Verification items for this drawing (mm, ordinates from the low corner). Round coordinates to 2 decimals unless told otherwise and drop trailing zeros. Loops run counter-clockwise (first coordinate to the right, second up) from the corner with the lowest first, then second, coordinate; pieces in that order, holes last. Notation, with made-up numbers: (31, 32.5) - (65, 32.5) arc R30 ccw to (65, 65.5) - close; hole circle Ø7 at (19.25, 17). An arc over 180 degrees is marked (long way). Put each result on its own line as item: value.
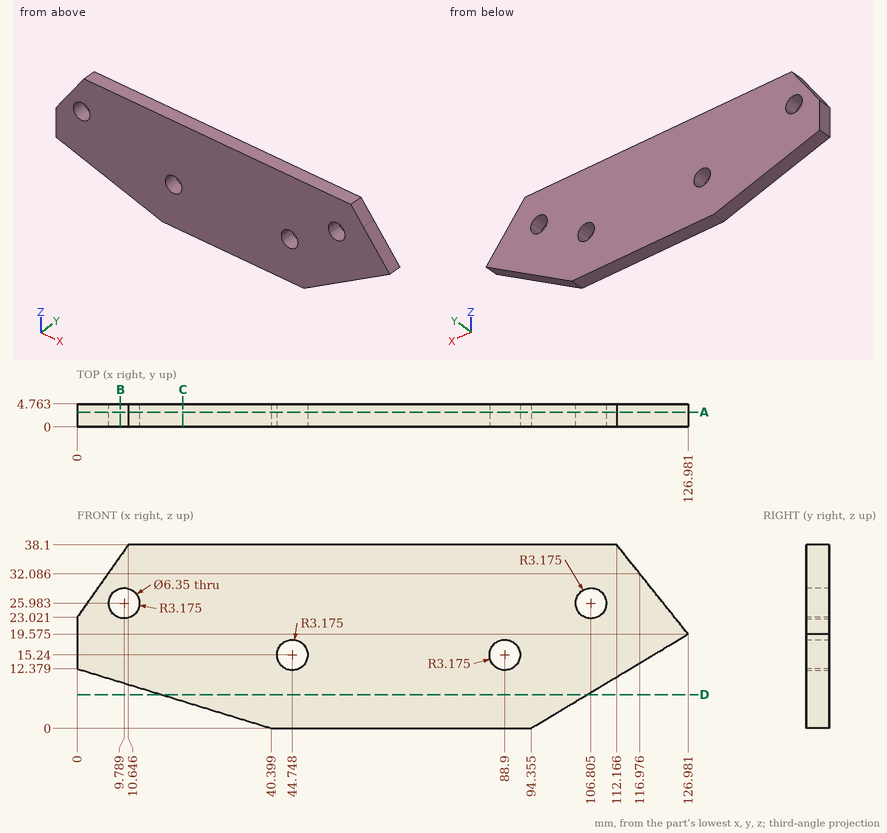
Item 1: Section check D-D on z = 7. Enter the section's corners in (x, y) (1 decimal).
Filled sheet:
outline: (17.6, 0) - (106, 0) - (106, 4.8) - (17.6, 4.8) - close
Item 2: Go/stop test with flat-tipped pins: pin 1 (1 mm diameter, centred on x = 34.5, y = 3.5, fed in from -Z) (1 decimal); pin 2 (4 mm diameter, centred on x = 9.79, z = 25.98, fed in from +Y); pin 3 (4 mm diameter, centred on x = 22.5, z = 22.5, fed in from -Y). Record where each tip stops, or that it passes through.
Filled sheet:
pin 1: z = 1.7
pin 2: through
pin 3: y = 0
Item 3: Section check C-C on x = 22. Enter the section's corners in (y, z).
Filled sheet:
outline: (0, 5.64) - (4.76, 5.64) - (4.76, 38.1) - (0, 38.1) - close
Item 4: Section check B-B on x = 9. Enter the section's corners in (y, z).
Filled sheet:
outline: (0, 9.62) - (4.76, 9.62) - (4.76, 22.91) - (0, 22.91) - close; (0, 29.06) - (4.76, 29.06) - (4.76, 35.77) - (0, 35.77) - close
Item 5: Section check A-A on y = 3.1. Count the separate pieces of the cut face and the enclosed holes in it, then the cut area to 3 significant figures.
Filled sheet:
separate pieces: 1
enclosed holes: 4
area: 3,920 mm²
Item 6: Thickness scan on line 1 (X direction, y = 2.3, z = 16) (1 decimal); line 2 (Z direction, x = 89, y = 0.35); line 3 (X direction, y = 2.3, z = 23.5) (1 decimal). Record the ranges inside material, lowest first. Write a range as from..to.
Filled sheet:
line 1: 0..41.7, 47.8..85.8, 92..121
line 2: 0..12.07, 18.41..38.1
line 3: 0.3..7.8, 11.8..104.8, 108.8..123.8
